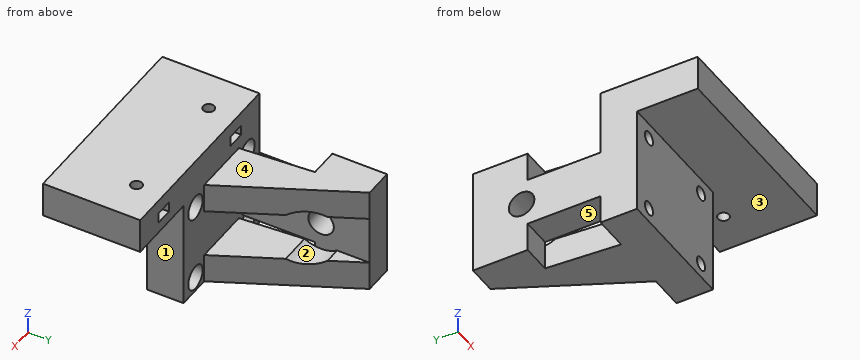
Autodesk Inventor part; units mm, degrees
ref_plane "YZ Plane" through (0, 0, 0) normal (1, 0, 0) x (0, 1, 0)
ref_plane "XZ Plane" through (0, 0, 0) normal (0, 1, 0) x (-1, 0, 0)
ref_plane "XY Plane" through (0, 0, 0) normal (0, 0, 1) x (1, 0, 0)
sketch "Sketch1" plane through (0, 0, 0) normal (0, 1, 0) x (-1, 0, 0)
  line L0 (-26.25, 22) -> (26.25, 22)
  line L1 (26.25, 22) -> (26.25, -22)
  line L2 (26.25, -22) -> (-26.25, -22)
  line L3 (-26.25, -22) -> (-26.25, 22)
  line L4 (-26.25, 22) -> (26.25, -22) construction
  line L5 (26.25, 22) -> (-26.25, -22) construction
  point P0 (0, 0)
  dimension "d0" = 44
  dimension "d1" = 52.5
extrude "Extrusion1" add sketch "Sketch1" along normal blind 67.5
sketch "Sketch2" plane through (0, 67.5, 0) normal (0, 1, 0) x (1, 0, 0)
  line L0 (18, -16) -> (-18, -16) construction
  line L1 (-18, -16) -> (-18, 16) construction
  line L2 (-18, 16) -> (18, 16) construction
  line L3 (18, 16) -> (18, -16) construction
  line L4 (18, -16) -> (-18, 16) construction
  line L5 (-18, -16) -> (18, 16) construction
  point P0 (0, 0)
  point P1 (-18, 16)
  dimension "d4" = 32
  dimension "d5" = 36
hole "Hole1" at (-18, 67.5, -16) at (-18, 67.5, 16) at (18, 67.5, 16) at (18, 67.5, -16) direction (0, -1, 0) diameter 5.6 end through all
sketch "Sketch3" plane through (-26.25, 0, -22) normal (-1, 0, 0) x (0, 0, 1)
  line L0 (0, 0) -> (44, 0)
  line L1 (44, 0) -> (44, 67.5)
  line L2 (0, 67.5) -> (44, 67.5)
  line L3 (0, 0) -> (0, 67.5)
  point P0 (22, 0)
  point P1 (22, 47.5)
  point P2 (22, 0)
  dimension "d13" = 47.5
hole "Hole2" at (-26.25, 47.5, 0) direction (1, 0, 0) diameter 10.5 end through all
sketch "Sketch4" plane through (0, 67.5, 0) normal (0, 1, 0) x (1, 0, 0)
  circle A0 centre (18, 16) radius 2.8
  circle A1 centre (18, -16) radius 2.8
  circle A2 centre (-18, -16) radius 2.8
  circle A3 centre (-18, 16) radius 2.8
  line L0 (26.25, 22) -> (-26.25, 22)
  line L1 (-26.25, 22) -> (-26.25, -22)
  line L2 (-26.25, -22) -> (26.25, -22)
  line L3 (26.25, -22) -> (26.25, 22)
  line L4 (26.25, 22) -> (-14.25, 22)
  line L5 (-14.25, 22) -> (-14.25, -22)
  line L6 (-14.25, -22) -> (26.25, -22)
  line L7 (26.25, -22) -> (26.25, 22)
  line L8 (-26.25, 22) -> (-14.25, 22)
  line L9 (-14.25, 22) -> (-14.25, 10)
  line L10 (-14.25, 10) -> (-26.25, 10)
  line L11 (-26.25, 10) -> (-26.25, 22)
  line L12 (-14.25, -22) -> (-26.25, -22)
  line L13 (-26.25, -22) -> (-26.25, -10)
  line L14 (-26.25, -10) -> (-14.25, -10)
  line L15 (-14.25, -10) -> (-14.25, -22)
  point P0 (0, 0)
  dimension "d21" = 12
  dimension "d22" = 6
  dimension "d23" = 6
  dimension "d24" = 6
extrude "Extrusion2" cut sketch "Sketch4" against normal blind 52.5 contours L3 L2 L5 L0 | L5 L10 L1 L0 | L2 L1 L14 L5
sketch "Sketch5" plane through (-26.25, 67.5, 10) normal (0, 0, 1) x (1, 0, 0)
  line L0 (0, 0) -> (12, 0)
  line L1 (0, -52.5) -> (0, 0)
  line L2 (0, -52.5) -> (12, -52.5)
  line L3 (12, 0) -> (12, -52.5)
  line L4 (52.5, -52.5) -> (0, -52.5)
  line L5 (11.05, -52.5) -> (5.45, -52.5)
  line L6 (8.25, -52.5) -> (8.25, 0) construction
  line L7 (12, -22.5) -> (14.25, -52.5)
  line L8 (12, 0) -> (38.25, -52.5)
  line L9 (47.05, -52.5) -> (41.45, -52.5)
  line L10 (44.25, -52.5) -> (44.25, -22.1018) construction
  line L11 (12, -22.5) -> (0, -22.5)
  line L12 (0, -22.5) -> (0, 0)
  line L13 (0, 0) -> (12, 0)
  line L14 (38.25, -52.5) -> (14.25, -52.5)
  point P0 (26.25, -67.5)
  dimension "d27" = 30
  dimension "d28" = 36
  dimension "d29" = 6
  dimension "d30" = 6
extrude "Extrusion3" add sketch "Sketch5" along normal up to surface (12 mm away) contours L0 L3 L11 L1 | L8 L4 L7 L3
sketch "Sketch6" plane through (0, 15, 0) normal (0, 1, 0) x (1, 0, 0)
  circle A0 centre (-18, -16) radius 2.8
  circle A1 centre (18, -16) radius 2.8
  circle A2 centre (18, 16) radius 2.8
  circle A3 centre (-18, 16) radius 2.8
  circle A4 centre (-18, 16) radius 2.8
  point P0 (0, 0)
hole "Hole3" at (-18, 15, 16) at (18, 15, -16) at (-18, 15, -16) at (18, 15, 16) direction (0, -1, 0) diameter 5.5 end through all counterbore diameter 10 counterbore depth 5.7
mirror "Mirror1" about plane through (0, 0, 0) normal (0, 0, 1) of "Extrusion3"
sketch "Sketch7" plane through (-14.25, 15, 10) normal (1, 0, 0) x (0, 0, -1)
  circle A0 centre (10, 32.5) radius 5.25
  circle A1 centre (10, 32.5) radius 12
  point P0 (10, -15)
  dimension "d40" = 24
extrude "Extrusion4" cut sketch "Sketch7" along normal through all contours A0 | A1
sketch "Sketch8" plane through (-26.25, 0, 22) normal (0, 0, 1) x (1, 0, 0)
  line L0 (52.5, 15) -> (38.25, 15)
  line L1 (12, 67.5) -> (38.25, 15)
  line L2 (0, 67.5) -> (12, 67.5)
  line L3 (0, 45) -> (0, 67.5)
  line L4 (12, 45) -> (0, 45)
  line L5 (14.25, 15) -> (12, 45)
  line L6 (14.25, 15) -> (0, 15)
  line L7 (0, 0) -> (0, 15)
  line L8 (0, 0) -> (52.5, 0)
  line L9 (52.5, 0) -> (52.5, 15)
  line L10 (14.25, 15) -> (38.25, 15)
  point P0 (26.25, 0)
extrude "Extrusion5" add sketch "Sketch8" along normal blind 15 contours L9 L8 L7 L6 L10 L0
sketch "Sketch9" plane through (0, 0, 0) normal (0, -1, 0) x (1, 0, 0)
  circle A0 centre (18, -16) radius 2.8
  circle A1 centre (18, 16) radius 2.8
  circle A2 centre (-18, 16) radius 2.8
  circle A3 centre (-18, -16) radius 2.8
  line L0 (26.25, -22) -> (-26.25, -22)
  line L1 (26.25, -22) -> (26.25, 37)
  line L2 (-26.25, 37) -> (26.25, 37)
  line L3 (-26.25, -22) -> (-26.25, 37)
  line L4 (-26.25, 22.5) -> (27.0192, 22.5)
  point P0 (0, 0)
  point P1 (26.25, 22.5)
  dimension "d45" = 14.5
extrude "Extrusion6" add sketch "Sketch9" along normal blind 25 contours L4 L3 L2 L1
sketch "Sketch10" plane through (26.25, 0, -22) normal (1, 0, 0) x (0, 0, -1)
  line L0 (0, 15) -> (-59, 15)
  line L1 (-59, 15) -> (-59, -25)
  line L2 (-44.5, -25) -> (-59, -25)
  line L3 (-44.5, 0) -> (-44.5, -25)
  line L4 (0, 0) -> (-44.5, 0)
  line L5 (0, 0) -> (0, 15)
  line L6 (-44.5, 0) -> (-44.5, 15)
  point P0 (-22, 0)
extrude "Extrusion7" add sketch "Sketch10" along normal blind 30 contours L6 L3 L2 L1 L0
sketch "Sketch11" plane through (-26.25, 0, 37) normal (0, 0, 1) x (1, 0, 0)
  line L0 (0, 15) -> (0, -25)
  line L1 (0, -25) -> (82.5, -25)
  line L2 (82.5, 15) -> (82.5, -25)
  line L3 (0, 15) -> (82.5, 15)
  line L4 (0, 15) -> (82.5, -25) construction
  line L5 (82.5, 15) -> (0, -25) construction
  line L6 (-31.1297, -30) -> (116.2871, -30) construction
  point P0 (26.25, 0)
  point P1 (16.25, 3.8)
  point P2 (66.25, 3.8)
  point P3 (41.25, -5)
  dimension "d50" = 50
  dimension "d51" = 25
  dimension "d52" = 5
  dimension "d53" = 33.8
hole "Hole4" at (-10, 3.8, 37) at (40, 3.8, 37) direction (0, 0, -1) diameter 4.6 depth 10
sketch "Sketch12" plane through (40, 3.8, 27) normal (0, 0, 1) x (1, 0, 0)
  circle A0 centre (0, 0) radius 2.3
  circle A1 centre (-50, 0) radius 2.3
  line L0 (-46.4, 2.0785) -> (-46.4, -2.0785)
  line L1 (-46.4, -2.0785) -> (-50, -4.1569)
  line L2 (-50, -4.1569) -> (-53.6, -2.0785)
  line L3 (-53.6, -2.0785) -> (-53.6, 2.0785)
  line L4 (-53.6, 2.0785) -> (-50, 4.1569)
  line L5 (-50, 4.1569) -> (-46.4, 2.0785)
  line L6 (0, 4.1569) -> (3.6, 2.0785)
  line L7 (3.6, 2.0785) -> (3.6, -2.0785)
  line L8 (3.6, -2.0785) -> (0, -4.1569)
  line L9 (0, -4.1569) -> (-3.6, -2.0785)
  line L10 (-3.6, -2.0785) -> (-3.6, 2.0785)
  line L11 (-3.6, 2.0785) -> (0, 4.1569)
  line L12 (-66.25, 11.2) -> (16.25, 11.2)
  line L13 (-53.6, 2.0785) -> (-53.6, 11.2)
  line L14 (-46.4, 2.0785) -> (-46.4, 11.2)
  line L15 (-3.6, 2.0785) -> (-3.6, 11.2)
  line L16 (3.6, 2.0785) -> (3.6, 11.2)
  point P0 (-40, -3.8)
  point P1 (-50, 0)
  dimension "d61" = 7.2
extrude "Extrusion8" cut sketch "Sketch12" along normal blind 4.2
sketch "Sketch13" plane through (-13.6, 1.7215, 27) normal (0, 0, 1) x (1, 0, 0)
  circle A0 centre (3.6, 2.0785) radius 2.3
  circle A1 centre (3.6, 2.0785) radius 2.3
  circle A2 centre (53.6, 2.0785) radius 2.3
  circle A3 centre (53.6, 2.0785) radius 2.3
  point P0 (13.6, -1.7215)
hole "Hole5" at (-10, 3.8, 27) at (40, 3.8, 27) direction (0, 0, -1) diameter 4.6 depth 5
equation "\"d23\" = d22"
equation "\"d24\" = d23"
equation "\"d30\" = d29"
properties part number "Part1_3DPrint"
Source: CAD feature listing. Evaluate the final solid. Frame: model axes, mm. Face numbers are marked on the shaded views. A direction names the side the tool comes from. Round coordinates to 2 decimals unless told otherwise and drop trailing zeros. Loops run counter-clockwise (first coordinate to the right, second up) from the corner with the lowest first, then second, coordinate; pieces in that order, holes last. Notation, with made-up numbers: M -25,29.5 L 29,29.5 A6 cw 29,40.5 Z; hole C 83.25,78.5 d5. An arc over 180 degrees is marked long. Use a Markdown table: item, result. Add a question column.
1. Line query: line 1 (Z direction, x = 18, y = 10.5); line 2 (X direction, y = 3.8, z = 32.95); line 3 (X direction, y = 13, z = 16). Output: solid intervals per line, ascending.
2. Contact query for flat-ended pins moving along their axis: P1, Ø5.5, axis at x = 40, y = 3.8, coming from the -Z side; P2, Ø12, axis at x = -15.5, z = -2.5, coming from the -Y side; P3, Ø5.5, axis at x = -10.5, y = 60.5, coming from the +Z side. Output: stop coordinate, or through.
3. Reachability of the marked faces 1, 2, 3, 4 and 5 from +Z, -Z, +X, -X, +Y, -Y: full face, straight path, thin tool, end or side. Return the list, or none.
4. Section query B-B on y = 47.5. Return the cut outline in (x, z), then the cut area to 3 significant figures.
5. Section query A-A on x = -18. Give the number of separate pieces and of enclosed holes in the cut face, then the cut area to 3 significant figures.
6. Section query C-C on z = 0. Return the cut outline in (x, y).
Reported:
| question | item | result |
|---|---|---|
| 1 | line 1 | z = -22 to -21, -11 to 11, 21 to 37 |
| 1 | line 2 | x = -26.25 to -12.3, -7.7 to 37.7, 42.3 to 56.25 |
| 1 | line 3 | x = -26.25 to -23, -13 to 13, 23 to 26.25 |
| 2 | P1 | stops at z = 22.5 |
| 2 | P2 | stops at y = 0 |
| 2 | P3 | stops at z = 22 |
| 3 | face 1 | -Z, +X, +Y, -Y |
| 3 | face 2 | +X |
| 3 | face 3 | -Z, +X, -Y |
| 3 | face 4 | +Z, +X, -X, +Y |
| 3 | face 5 | -Z, -X |
| 4 | outline | M -26.25,-22 L -4.25,-22 L -4.25,-12 L -14.25,-12 L -14.25,-5.25 L -26.25,-5.25 Z; M -26.25,5.25 L -14.25,5.25 L -14.25,12 L -4.25,12 L -4.25,22 L -26.25,22 Z |
| 4 | area | 602 mm² |
| 5 | separate pieces | 3 |
| 5 | enclosed holes | 1 |
| 5 | area | 2,530 mm² |
| 6 | outline | M -26.25,0 L 26.25,0 L 26.25,15 L -14.25,15 L -14.25,42.25 L -26.25,42.25 Z; M -26.25,52.75 L -14.25,52.75 L -14.25,67.5 L -26.25,67.5 Z |
